The listing builds one solid part. Answer for the finished solid, in the listing's coordinates (mm). A direction names the side the tool comes from. Give positions to 0.01 mm unless a question says otherwise; leave off trailing zeros. Order: outer loops, then holes, each group sorted by start corner. A loop starts at its lowest first (then second) coordinate and runs counter-clockwise, first axis right, second up. Notation, with made-up numbers: (53, 37) -> (112, 37) arc R29 cw to (112, 67) -> close; hole circle Ø11 at (10.25, -5.75). An arc over 180 degrees is marked (long way). One line per question, with ' | ' between items. Start each with the question number.
```python
from build123d import *

# Parameters (mm, degrees)
F1_DEPTH = 50.8


with BuildPart() as f1:
    # F0 (on Right) → F1 (new body)
    with BuildSketch(Plane.YZ):
        Polygon((0, 58.321822), (0, 0), (41.221242, 28.256854), (114.869855, -45.376718), (68.702079, 31.017145), (135.755301, 21.60695), (47.816634, 65.576285), (10.442711, 127.418935), (0, 85.152954), (-78.595169, 103.396483), align=None)
    extrude(amount=-F1_DEPTH)


solid = f1.part
```
(1) Determine the mould class of faces 1 (the face through (0, 28, 48)), 2 (the face through (-25.044, 101.759, 26.378)), 3 (the face through (-25.044, 77.53, -8.044)) for opening direction Z: pulls with the +Z half, pulls with the -Z half, needs draft (parallel to the pull), parting line crosses it, or undercut.
(2) The part is cut by section A-A on z = 88.5. Determine the outline of the cut face in (x, y).
(3) The part is cut by section B-B on y = 75.5. Determine the outline of the cut face in (x, z).
(4) For faces 4 (the face through (-25.044, -38.747, 94.147)), 5 (the face through (-25.04, 20.32, 13.93)), 6 (the face through (-25, 0, 30)), determine the directions among +Z, -Z, +X, -X, +Y, -Y from which every point of the face is accessible in a straight line to the end or side of a thin tool.
(5) Consider line 1 (Y direction, x = -12, z = 1); line 2 (Y direction, x = -38, z = 1.5); line 3 (Z direction, x = -15.5, y = 82). Determine where each line is inside the solid, lowest interval first.
(6) The part is cut by section C-C on x = -35. Determine the outline of the cut face in (y, z), plus the area to 3 significant figures.
(7) The part is cut by section D-D on z = 37. Determine the outline of the cut face in (x, y), plus the area to 3 significant figures.
(8) Given P1, Ø1.5, axis at x = -37, z = 73, coming from the +Y side; P2, Ø4, axis at x = -38, z = 63.5, coming from the -Y side; P3, Ø1, axis at x = -40.5, y = -32, coming from the -Z side, each flat-ended and moving along its own axis, determine where each tip first touches the part or whether it passes through.
Result sheet:
1) face 1: needs draft | face 2: undercut | face 3: pulls with the -Z half
2) outline: (-50.8, -52.62) -> (0, -52.62) -> (0, -14.42) -> (-50.8, -14.42) -> close; (-50.8, 0.83) -> (0, 0.83) -> (0, 33.96) -> (-50.8, 33.96) -> close
3) outline: (-50.8, -6.01) -> (0, -6.01) -> (0, 19.77) -> (-50.8, 19.77) -> close; (-50.8, 30.06) -> (0, 30.06) -> (0, 51.73) -> (-50.8, 51.73) -> close
4) face 4: +Z, +X, -X | face 5: -Z, +X, -X | face 6: -Z, +X, -X, -Y
5) line 1: y = 0 to 1.46, 68.48 to 86.84 | line 2: y = 0 to 2.19, 67.98 to 86.54 | line 3: z = -12.51 to 9.01, 29.15 to 48.48
6) outline: (-78.6, 103.4) -> (0, 58.32) -> (0, 0) -> (41.22, 28.26) -> (114.87, -45.38) -> (68.7, 31.02) -> (135.76, 21.61) -> (47.82, 65.58) -> (10.44, 127.42) -> (0, 85.15) -> close | area: 7,560 mm^2
7) outline: (-50.8, 0) -> (0, 0) -> (0, 104.97) -> (-50.8, 104.97) -> close | area: 5,330 mm^2
8) P1: stops at y = 43.78 | P2: stops at y = -12.52 | P3: stops at z = 76.39
